```python
from build123d import *
from OCP.BRepFilletAPI import BRepFilletAPI_MakeChamfer

# Parameters (mm, degrees)
SKETCH1_W           = 140.4
SKETCH1_H           = 110.4
BOSS_EXTRUDE1_DEPTH = 30
SHELL1_T            = -3.5
SKETCH2_W           = 140.4
SKETCH2_H           = 10.4
BOSS_EXTRUDE2_DEPTH = 5
CUT_EXTRUDE3_DEPTH  = 5
SKETCH5_W           = 12
SKETCH5_H           = 19.4
BOSS_EXTRUDE3_DEPTH = 24
CHAMFER1_SIZE       = 45
CHAMFER1_SIZE2      = 16.378660542
CHAMFER3_SIZE       = 5
BOSS_EXTRUDE5_DEPTH = 5


with BuildPart() as part:
    # Sketch1 → Boss-Extrude1 (new body)
    with BuildSketch(Plane(origin=(0, 0, 0), x_dir=(1, 0, 0), z_dir=(0, 1, 0))):
        Rectangle(SKETCH1_W, SKETCH1_H)
    extrude(amount=-BOSS_EXTRUDE1_DEPTH)

    # Shell1
    shell1_openings = [part.faces().sort_by_distance(p)[0] for p in [
        (0, 0, 0),
    ]]
    offset(amount=SHELL1_T, openings=shell1_openings, kind=Kind.INTERSECTION)

    # Sketch2 → Boss-Extrude2 (add)
    with BuildSketch(Plane(origin=(0, 0, 0), x_dir=(1, 0, 0), z_dir=(0, 1, 0))):
        with Locations((0, -50)):
            Rectangle(SKETCH2_W, SKETCH2_H)
    extrude(amount=BOSS_EXTRUDE2_DEPTH)

    # Sketch6 → Cut-Extrude3 (cut)
    with BuildSketch(Plane.ZY.offset(-66.7)):
        with BuildLine():
            Line((-4.4, -3.1), (4.4, -3.1))
            ThreePointArc((4.4, -3.1), (5.9, -4.6), (4.4, -6.1))
            Line((4.4, -6.1), (-4.4, -6.1))
            ThreePointArc((-4.4, -6.1), (-5.9, -4.6), (-4.4, -3.1))
        make_face()
    extrude(amount=-CUT_EXTRUDE3_DEPTH, mode=Mode.SUBTRACT)

    # Sketch5 → Boss-Extrude3 (add)
    with BuildSketch(Plane.ZY.offset(-66.7)):
        with Locations((0, -16.8)):
            Rectangle(SKETCH5_W, SKETCH5_H)
    extrude(amount=BOSS_EXTRUDE3_DEPTH)

    # Chamfer1: one chamfer whose edges measure the first distance from different faces: ONE call of the kernel's chamfer builder (chamfer() names one face for all edges)
    chamfer1_edges_1 = [part.edges().sort_by_distance(p)[0] for p in [
        (0, -26.5, 51.7),
    ]]
    chamfer1_side_1 = [part.faces().sort_by_distance(p)[0] for p in [
        (-1.166452928, -26.5, 0),
    ]]
    chamfer1_edges_2 = [part.edges().sort_by_distance(p)[0] for p in [
        (0, -30, 55.2),
    ]]
    chamfer1_side_2 = [part.faces().sort_by_distance(p)[0] for p in [
        (0, -30, 0),
    ]]
    chamfer1 = BRepFilletAPI_MakeChamfer(part.part.solid().wrapped)
    for e in chamfer1_edges_1:
        chamfer1.Add(CHAMFER1_SIZE, CHAMFER1_SIZE2, e.wrapped, chamfer1_side_1[0].wrapped)  # the first distance lies on this face
    for e in chamfer1_edges_2:
        chamfer1.Add(CHAMFER1_SIZE, CHAMFER1_SIZE2, e.wrapped, chamfer1_side_2[0].wrapped)  # the first distance lies on this face
    add(Compound.cast(chamfer1.Shape()), mode=Mode.REPLACE)

    # Chamfer3
    chamfer3_edges = [part.edges().sort_by_distance(p)[0] for p in [
        (-70.2, -30, -22.5),
        (-70.2, -15, -55.2),
        (70.2, -15, -55.2),
        (70.2, -4.310669729, 55.2),
        (-70.2, -4.310669729, 55.2),
        (70.2, -30, -22.5),
        (0, -30, -55.2),
    ]]
    chamfer(chamfer3_edges, length=CHAMFER3_SIZE)

    # Sketch10 → Boss-Extrude5 (add)
    with BuildSketch(Plane(origin=(65.2, 0, 0), x_dir=(0, 0, 1), z_dir=(1, 0, 0))):
        Polygon((-50.2, 30), (10.2, 30), (-50.2, 51.98380215), align=None)
    boss_extrude5 = extrude(amount=-BOSS_EXTRUDE5_DEPTH)

    # Mirror1: Boss-Extrude5 across plane
    add(boss_extrude5.mirror(Plane(origin=(0, 0, 0), x_dir=(0, 0, 1), z_dir=(1, 0, 0))))


solid = part.part
```
Work out the finished part from the listing and answer in its coordinate system (mm). A direction names the side the tool comes from. Give positions to 0.01 mm unless a question says otherwise; leave off trailing zeros. Order: outer loops, then holes, each group sorted by start corner. A loop starts at its lowest first (then second) coordinate and runs counter-clockwise, first axis right, second up. Notation, with made-up numbers: (88, -6) - (103, -6) arc R15 cw to (103, 15) - close; hole circle Ø10 at (-3.5, -8.75). An arc over 180 degrees is marked (long way). One line per item, written item: value. Start each with the question number.
1. Each of these flat-tipped pins is pushed along its axis until it touches: pin 1 Ø1.8 at (x, z) = (68, 1) entering from +Y; pin 2 Ø1.5 at (x, z) = (42, 30) entering from +Y; pin 3 Ø2.5 at (x, y) = (18.5, 3.5) entering from -Z; pin 4 Ø10 at (x, y) = (26.5, -39) entering from -Z. Where does it stop, or does it pass through?
2. Which of the six approach directions +Z, -Z, +X, -X, +Y, -Y give full straight-line access (tool end or side, diameter ignored) to faces 1 (the face through (-1, 2, 44.8)), 2 (the face through (68.4, -4.6, -5.9)), 3 (the face through (60.2, -36, -34)), 4 (the face through (-63, -41, -50.2))?
3. For a pull along Z with two mould halves and no side action, classify faces 5 (the face through (55, -17, 6)), 6 (the face through (-1, -30, -20)), 7 (the face through (-66.8, -26.5, -52.1)), 8 (the face through (-1, 0, 48)) as released by +Z, released by -Z, zero draft, split by the parting line, or undercut.
4. Section A-A, the plane y = -4.6 is taken. Write down the section's boundary in (x, z), then the cut area to 3 significant figures.
5. Consider line 1 (X direction, y = -13, z = 21.5); line 2 (Z direction, x = -17, y = -5.5); line 3 (Y direction, x = -14, z = -20). Determine where each line is inside the solid, lowest interval first.
6. Section C-C, the plane y = -22 is taken. Write down the section's boundary in (x, z), then the cut area to 3 significant figures.
7. Section B-B, the plane x = -45.5 is taken. Write down the section's boundary in (y, z).
8. Section D-D, the plane z = 33.5 is taken. Write down the section's boundary in (x, y).
Filled sheet:
1. pin 1: y = 0
1. pin 2: y = -17.75
1. pin 3: z = 44.8
1. pin 4: through
2. face 1: -Z, +X, -X, +Y
2. face 2: +X
2. face 3: +Z, -Z, -Y
2. face 4: -Z, +X, -X, -Y
3. face 5: undercut
3. face 6: zero draft
3. face 7: released by -Z
3. face 8: undercut
4. outline: (-70.2, -50.2) - (-65.2, -55.2) - (65.2, -55.2) - (70.2, -50.2) - (70.2, -5.9) - (66.7, -5.9) - (66.7, -51.7) - (-66.7, -51.7) - (-66.7, 51.7) - (66.7, 51.7) - (66.7, 5.9) - (70.2, 5.9) - (70.2, 50.2) - (65.2, 55.2) - (-65.2, 55.2) - (-70.2, 50.2) - close
4. area: 1,620 mm²
5. line 1: -70.2 to -66.7, 66.7 to 70.2
5. line 2: -55.2 to -51.7, 51.7 to 55.2
5. line 3: -30 to -26.5
6. outline: (-70.2, -50.2) - (-65.2, -55.2) - (65.2, -55.2) - (70.2, -50.2) - (70.2, 32.18) - (-70.2, 32.18) - close; hole (-66.7, -51.7) - (66.7, -51.7) - (66.7, -6) - (42.7, -6) - (42.7, 6) - (66.7, 6) - (66.7, 19.06) - (-66.7, 19.06) - close
6. area: 3,090 mm²
7. outline: (-30, -50.2) - (-25, -55.2) - (0, -55.2) - (0, -51.7) - (-26.5, -51.7) - (-26.5, 6.7) - (-10.12, 51.7) - (0, 51.7) - (0, 44.8) - (5, 44.8) - (5, 55.2) - (-13.62, 55.2) - (-30, 10.2) - close
8. outline: (-70.2, -21.52) - (70.2, -21.52) - (70.2, 0) - (66.7, 0) - (66.7, -16.75) - (-66.7, -16.75) - (-66.7, 0) - (-70.2, 0) - close
